Verification items for the finished model (mm, model axes). Coordinates: 2 decimals unless noted, no trailing zeros. Order: outer loops, then holes, each group sorted by start corner. A loop starts at its lowest first (then second) coordinate and runs counter-clockwise, first axis right, second up. Notation, with made-up numbers: (63, 27.25) -> (119, 27.25) arc R24 ccw to (119, 62.25) -> close; hole circle Ø6 at (85, 2.5). An arc over 180 degrees is marked (long way). Write item = value, one per line. Start each with the question number.
Autodesk Inventor part; units mm, degrees
ref_plane "YZ Plane" through (0, 0, 0) normal (1, 0, 0) x (0, 1, 0)
ref_plane "XZ Plane" through (0, 0, 0) normal (0, 1, 0) x (-1, 0, 0)
ref_plane "XY Plane" through (0, 0, 0) normal (0, 0, 1) x (1, 0, 0)
sketch "Sketch1" plane through (0, 0, 0) normal (0, 0, 1) x (1, 0, 0)
  line L0 (-70, 40) -> (70, 40) construction
  line L1 (70, 40) -> (70, -40) construction
  line L2 (70, -40) -> (-70, -40) construction
  line L3 (-70, -40) -> (-70, 40) construction
  line L4 (90, 60) -> (-90, 60)
  line L5 (-90, 60) -> (-90, -60)
  line L6 (-90, -60) -> (90, -60)
  line L7 (90, -60) -> (90, 60)
  circle A0 centre (-80, -50) radius 3
  circle A1 centre (80, 50) radius 3
  circle A2 centre (0, -50) radius 3
  circle A3 centre (80, -50) radius 3
  circle A4 centre (-80, 50) radius 3
  line L8 (0, 60) -> (0, -60) construction
  line L9 (-90, 0) -> (90, 0) construction
  circle A5 centre (-35, 50) radius 3
  circle A6 centre (35, 50) radius 3
  circle A7 centre (0, 22.5) radius 2.15
  circle A8 centre (0, -27.5) radius 2.15
  circle A9 centre (37, 0) radius 2.15
  circle A10 centre (-37, 0) radius 2.15
  point P0 (0, 0)
  point P1 (-70, 0)
  point P2 (0, 40)
  point P3 (0, 0)
  dimension "d0" = 140
  dimension "d1" = 80
  dimension "d2" = 20
  dimension "d3" = 6
  dimension "d4" = 10
  dimension "d5" = 10
  dimension "d8" = 35
  dimension "d9" = 4.3
  dimension "d10" = 74
  dimension "d11" = 50
  dimension "d12" = 27.5
extrude "Extrusion1" add sketch "Sketch1" along normal blind 6
properties part number "top"
Item 1: Section check A-A (y = 50). Record the boundary of the cut face in (x, z), then the cut area to 3 significant figures.
Item 2: Thickness scan on line 1 (Y direction, x = -80, z = 1.4); line 2 (X direction, y = -50.5, z = 3.05); line 3 (Y direction, x = 37, z = 3.45). Record the ranges inside material, lowest first.
Item 3: Mould release check, pull along Y, two halves, no side actions. Record for faces 1 (the flat face through (-90, 1, 3)), 2 (the flat face through (1, 60, 3)), 3 (the cylindrical face through (-82.21, -52.03, 2.96)): pulls with the +Y half, pulls with the -Y half, needs draft (parallel to the pull), parting line crosses it, or undercut.
Item 4: Section check B-B (x = 79). Record the boundary of the cut face in (y, z), then the cut area to 3 significant figures.
Filled sheet:
q1.outline = (-90, 0) -> (-83, 0) -> (-83, 6) -> (-90, 6) -> close; (-77, 0) -> (-38, 0) -> (-38, 6) -> (-77, 6) -> close; (-32, 0) -> (32, 0) -> (32, 6) -> (-32, 6) -> close; (38, 0) -> (77, 0) -> (77, 6) -> (38, 6) -> close; (83, 0) -> (90, 0) -> (90, 6) -> (83, 6) -> close
q1.area = 936 mm^2
q2.line_1 = -60 to -53, -47 to 47, 53 to 60
q2.line_2 = -90 to -82.96, -77.04 to -2.96, 2.96 to 77.04, 82.96 to 90
q2.line_3 = -60 to -2.15, 2.15 to 47.76, 52.24 to 60
q3.face_1 = needs draft
q3.face_2 = pulls with the +Y half
q3.face_3 = undercut
q4.outline = (-60, 0) -> (-52.83, 0) -> (-52.83, 6) -> (-60, 6) -> close; (-47.17, 0) -> (47.17, 0) -> (47.17, 6) -> (-47.17, 6) -> close; (52.83, 0) -> (60, 0) -> (60, 6) -> (52.83, 6) -> close
q4.area = 652 mm^2
